```python
from build123d import *

# Parameters (mm, degrees)
SKETCH_1_W      = 3.75
SKETCH_1_H      = 3.75
EXTRUDE_1_DEPTH = 250


with BuildPart() as part:
    # 草图1 → 凸台-拉伸1 (new body)
    with BuildSketch(Plane.XY):
        with BuildLine():
            Line((-5.2, -15), (-5.2, -14))
            Line((-5.2, -14), (-4.1, -14))
            Line((-4.1, -14), (-4.1, -13))
            Line((-4.1, -13), (-8.25, -13))
            Line((-8.25, -13), (-8.25, -9.664213562))
            Line((-8.25, -9.664213562), (-4.385786438, -5.8))
            Line((-4.385786438, -5.8), (4.385786438, -5.8))
            Line((4.385786438, -5.8), (8.25, -9.664213562))
            Line((8.25, -9.664213562), (8.25, -13))
            Line((8.25, -13), (4.1, -13))
            Line((4.1, -13), (4.1, -14))
            Line((4.1, -14), (5.2, -14))
            Line((5.2, -14), (5.2, -15))
            Line((5.2, -15), (12.5, -15))
            ThreePointArc((12.5, -15), (14.267766953, -14.267766953), (15, -12.5))
            Line((15, -12.5), (15, -5.2))
            Line((15, -5.2), (14, -5.2))
            Line((14, -5.2), (14, -4.1))
            Line((14, -4.1), (13, -4.1))
            Line((13, -4.1), (13, -8.25))
            Line((13, -8.25), (9.664213562, -8.25))
            Line((9.664213562, -8.25), (5.8, -4.385786438))
            Line((5.8, -4.385786438), (5.8, 4.385786438))
            Line((5.8, 4.385786438), (9.664213562, 8.25))
            Line((9.664213562, 8.25), (13, 8.25))
            Line((13, 8.25), (13, 4.1))
            Line((13, 4.1), (14, 4.1))
            Line((14, 4.1), (14, 5.2))
            Line((14, 5.2), (15, 5.2))
            Line((15, 5.2), (15, 12.5))
            ThreePointArc((15, 12.5), (14.267766953, 14.267766953), (12.5, 15))
            Line((12.5, 15), (5.2, 15))
            Line((5.2, 15), (5.2, 14))
            Line((5.2, 14), (4.1, 14))
            Line((4.1, 14), (4.1, 13))
            Line((4.1, 13), (8.25, 13))
            Line((8.25, 13), (8.25, 9.664213562))
            Line((8.25, 9.664213562), (4.385786438, 5.8))
            Line((4.385786438, 5.8), (-4.385786438, 5.8))
            Line((-4.385786438, 5.8), (-8.25, 9.664213562))
            Line((-8.25, 9.664213562), (-8.25, 13))
            Line((-8.25, 13), (-4.1, 13))
            Line((-4.1, 13), (-4.1, 14))
            Line((-4.1, 14), (-5.2, 14))
            Line((-5.2, 14), (-5.2, 15))
            Line((-5.2, 15), (-12.5, 15))
            ThreePointArc((-12.5, 15), (-14.267766953, 14.267766953), (-15, 12.5))
            Line((-15, 12.5), (-15, 5.2))
            Line((-15, 5.2), (-14, 5.2))
            Line((-14, 5.2), (-14, 4.1))
            Line((-14, 4.1), (-13, 4.1))
            Line((-13, 4.1), (-13, 8.25))
            Line((-13, 8.25), (-9.664213562, 8.25))
            Line((-9.664213562, 8.25), (-5.8, 4.385786438))
            Line((-5.8, 4.385786438), (-5.8, -4.385786438))
            Line((-5.8, -4.385786438), (-9.664213562, -8.25))
            Line((-9.664213562, -8.25), (-13, -8.25))
            Line((-13, -8.25), (-13, -4.1))
            Line((-13, -4.1), (-14, -4.1))
            Line((-14, -4.1), (-14, -5.2))
            Line((-14, -5.2), (-15, -5.2))
            Line((-15, -5.2), (-15, -12.5))
            ThreePointArc((-15, -12.5), (-14.267766953, -14.267766953), (-12.5, -15))
            Line((-12.5, -15), (-5.2, -15))
        make_face()
        with Locations((11.125, 11.125)):
            Rectangle(SKETCH_1_W, SKETCH_1_H, mode=Mode.SUBTRACT)
        with Locations((-11.125, 11.125)):
            Rectangle(SKETCH_1_W, SKETCH_1_H, mode=Mode.SUBTRACT)
        with Locations((-11.125, -11.125)):
            Rectangle(SKETCH_1_W, SKETCH_1_H, mode=Mode.SUBTRACT)
        with Locations((11.125, -11.125)):
            Rectangle(SKETCH_1_W, SKETCH_1_H, mode=Mode.SUBTRACT)
        with BuildLine():
            Line((-3.712310601, 4.772970773), (-1.814611278, 2.87527145))
            ThreePointArc((-1.814611278, 2.87527145), (0, 3.4), (1.814611278, 2.87527145))
            Line((1.814611278, 2.87527145), (3.712310601, 4.772970773))
            ThreePointArc((3.712310601, 4.772970773), (4.772970773, 4.772970773), (4.772970773, 3.712310601))
            Line((4.772970773, 3.712310601), (2.87527145, 1.814611278))
            ThreePointArc((2.87527145, 1.814611278), (3.4, 0), (2.87527145, -1.814611278))
            Line((2.87527145, -1.814611278), (4.772970773, -3.712310601))
            ThreePointArc((4.772970773, -3.712310601), (4.772970773, -4.772970773), (3.712310601, -4.772970773))
            Line((3.712310601, -4.772970773), (1.814611278, -2.87527145))
            ThreePointArc((1.814611278, -2.87527145), (0, -3.4), (-1.814611278, -2.87527145))
            Line((-1.814611278, -2.87527145), (-3.712310601, -4.772970773))
            ThreePointArc((-3.712310601, -4.772970773), (-4.772970773, -4.772970773), (-4.772970773, -3.712310601))
            Line((-4.772970773, -3.712310601), (-2.87527145, -1.814611278))
            ThreePointArc((-2.87527145, -1.814611278), (-3.4, 0), (-2.87527145, 1.814611278))
            Line((-2.87527145, 1.814611278), (-4.772970773, 3.712310601))
            ThreePointArc((-4.772970773, 3.712310601), (-4.772970773, 4.772970773), (-3.712310601, 4.772970773))
        make_face(mode=Mode.SUBTRACT)
    extrude(amount=EXTRUDE_1_DEPTH)


solid = part.part
```
Model file for the job. Use its own axes, mm. A direction names the side the tool comes from. Coordinates: 2 decimals unless noted, no trailing zeros. Answer as a JSON object with one key per item and string values. Group by question number.
1) Flat gauge pins, fed straight in: pin 1 (6 mm diameter, centred on x = 11, y = -8, fed in from -Z); pin 2 (0.5 mm diameter, centred on y = -14.5, z = 121.5, fed in from -X); pin 3 (4.5 mm diameter, centred on y = 0.5, z = 152.5, fed in from +X); pin 4 (0.8 mm diameter, centred on y = 14.5, z = 95, fed in from +X). Where does each tip first touch, or does it go through?
2) Drill centre lines: L1, parallel to X at y = 11.5, z = 33; L2, parallel to Y at x = -12.75, z = 42.5; L3, parallel to Y at x = -0.5, z = 203.5. Where is each one in solid material? Low to high.
3) Cut at A-A, the plane z = 213.5. Count the separate pieces of the cut face and the enclosed holes in it, then the cut area to 3 significant figures.
4) Pull direction Y, two halves, no side cores. Call faces 3 (the face through (15, -9, 123)), 4 (the face through (9, 15, 123)), 5 (the face through (7.705, 6.291, 123.25)): +Y half, -Y half, draft (parallel to the pull), parting line (faces both ways), or undercut.
5) Which spindle directions (+Z, -Z, +X, -X, +Y, -Y) get a long thin tool onto all of the face, cutting with end or side? Do faces 1 (the face through (-9, -15, 123)), 2 (the face through (13, 6, 123)). Say none if no direction does.
Check values:
{
 "1": {"pin 1": "stops at z = 0", "pin 2": "stops at x = -14.29", "pin 3": "stops at x = 5.8", "pin 4": "stops at x = 14.42"},
 "2": {"L1": "x = -15 to -13, -9.25 to -8.25, 8.25 to 9.25, 13 to 15", "L2": "y = -14.99 to -13, -9.25 to -8.25, 8.25 to 9.25, 13 to 14.99", "L3": "y = -5.8 to -3.36, 3.36 to 5.8"},
 "3": {"separate pieces": "1", "enclosed holes": "5", "area": "293 mm²"},
 "4": {"face 3": "draft", "face 4": "+Y half", "face 5": "undercut"},
 "5": {"face 1": "+Z, -Z, +X, -X, -Y", "face 2": "+Z, -Z"}
}
